Source: CAD feature listing. Evaluate the final solid. Frame: model axes, mm. Give positions to 0.01 mm unless a question says otherwise; leave off trailing zeros. Write each loop counter-clockwise with the first axis right and the second up, starting at its lowest first coordinate (ties: lowest second). Pieces come first, ordered by that corner, then holes. Notation, with made-up numbers: M 56,-5.75 L 114,-5.75 A17 ccw 114,6.25 Z; hole C 63,11.25 d11. An arc over 180 degrees is marked long. Answer as a JSON object with one key per item and string values. Group by question number.
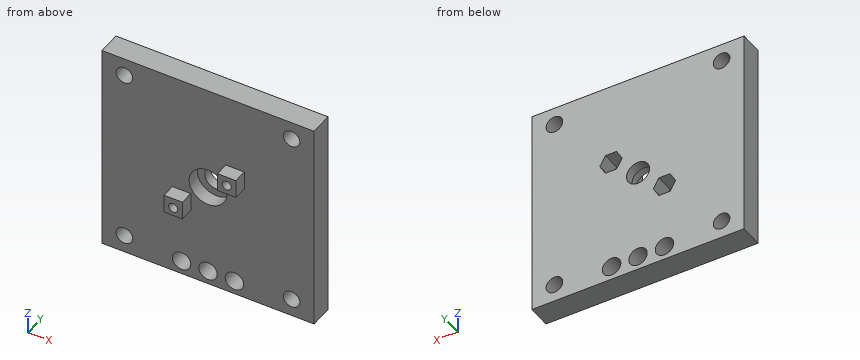
```python
from build123d import *

# Parameters (mm, degrees)
SKETCH2_W           = 46
SKETCH2_H           = 46
BOSS_EXTRUDE1_DEPTH = 5
SKETCH3_R           = 1.8
SKETCH3_R_2         = 2.5
CUT_EXTRUDE1_DEPTH  = 5
SKETCH4_R           = 4.1
CUT_EXTRUDE2_DEPTH  = 3
SKETCH5_W           = 4
SKETCH5_H           = 4
BOSS_EXTRUDE2_DEPTH = 3
SKETCH6_R           = 1
CUT_EXTRUDE3_DEPTH  = 9
CUT_EXTRUDE5_DEPTH  = 4
SKETCH9_R           = 2
CUT_EXTRUDE6_DEPTH  = 6


with BuildPart() as part:
    # Sketch2 → Boss-Extrude1 (new body)
    with BuildSketch(Plane(origin=(0, 0, 0), x_dir=(1, 0, 0), z_dir=(0, 1, 0))):
        Rectangle(SKETCH2_W, SKETCH2_H)
    extrude(amount=BOSS_EXTRUDE1_DEPTH)

    # Sketch3 → Cut-Extrude1 (cut)
    with BuildSketch(Plane(origin=(0, 0, 0), x_dir=(1, 0, 0), z_dir=(0, 1, 0))):
        with Locations((-18.12, 19.125)):
            Circle(SKETCH3_R)
        with Locations((18.12, 19.125)):
            Circle(SKETCH3_R)
        with Locations((18.12, -19.125)):
            Circle(SKETCH3_R)
        with Locations((-18.12, -19.125)):
            Circle(SKETCH3_R)
        Circle(SKETCH3_R_2)
    extrude(amount=CUT_EXTRUDE1_DEPTH, mode=Mode.SUBTRACT)

    # Sketch4 → Cut-Extrude2 (cut)
    with BuildSketch(Plane(origin=(0, 0, 0), x_dir=(1, 0, 0), z_dir=(0, 1, 0))):
        Circle(SKETCH4_R)
    extrude(amount=CUT_EXTRUDE2_DEPTH, mode=Mode.SUBTRACT)

    # Sketch5 → Boss-Extrude2 (add)
    with BuildSketch(Plane(origin=(0, 0, 0), x_dir=(1, 0, 0), z_dir=(0, 1, 0))):
        with Locations((-5.7330026, 5.06948708)):
            Rectangle(SKETCH5_W, SKETCH5_H)
        with Locations((5.862376563, -4.939727226)):
            Rectangle(SKETCH5_W, SKETCH5_H)
    extrude(amount=-BOSS_EXTRUDE2_DEPTH)

    # Sketch6 → Cut-Extrude3 (cut, through all)
    with BuildSketch(Plane(origin=(0, -3, 0), x_dir=(-1, 0, 0), z_dir=(0, -1, 0))):
        with Locations((5.7330026, 5.230811807)):
            Circle(SKETCH6_R)
        with Locations((-5.862376563, -4.939727226)):
            Circle(SKETCH6_R)
    extrude(amount=-CUT_EXTRUDE3_DEPTH, mode=Mode.SUBTRACT)

    # Sketch8 → Cut-Extrude5 (cut)
    with BuildSketch(Plane(origin=(0, 5, 0), x_dir=(1, 0, 0), z_dir=(0, 1, 0))):
        Polygon((8.287247693, -4.939727226), (7.074812128, -2.839727226), (4.649940998, -2.839727226), (3.437505432, -4.939727226), (4.649940998, -7.039727226), (7.074812128, -7.039727226), align=None)
        Polygon((-3.30813147, 5.230811807), (-4.520567035, 7.330811807), (-6.945438166, 7.330811807), (-8.157873731, 5.230811807), (-6.945438166, 3.130811807), (-4.520567035, 3.130811807), align=None)
    extrude(amount=-CUT_EXTRUDE5_DEPTH, mode=Mode.SUBTRACT)

    # Sketch9 → Cut-Extrude6 (cut, through all)
    with BuildSketch(Plane(origin=(0, 0, 0), x_dir=(1, 0, 0), z_dir=(0, 1, 0))):
        with Locations((-5.7330026, 20)):
            Circle(SKETCH9_R)
        with Locations((5.73, 20)):
            Circle(SKETCH9_R)
        with Locations((0, 20)):
            Circle(SKETCH9_R)
    extrude(amount=CUT_EXTRUDE6_DEPTH, mode=Mode.SUBTRACT)


solid = part.part
```
(1) Section D-D, the plane y = 2.25. State how many separate pieces and enclosed holes the cut face has, plus the area to 3 significant figures.
(2) Section C-C, the plane z = -20. Return loops of the section in (x, y), plus the area to 3 significant figures.
(3) Section A-A, the plane y = -1.25. Return loops of the section in (x, z), plus the area to 3 significant figures.
(4) Ray query, L1, parallel to Z at x = 0, y = 3.65; L2, parallel to Z at x = 18.12, y = 1.8 (3 decimals); L3, parallel to X at y = 4.5, z = -20.5. Return the intervals inside material, ascending. Write a range as [from, to].
(5) Section B-B, the plane x = 18.12. Return loops of the section in (y, z) (3 decimals), plus the area to 3 significant figures.
(6) Contact query for flat-ended pins moving along their axis: pin 1 Ø6 at (x, z) = (0, 0) entering from -Y; pin 2 Ø14 at (x, z) = (4.5, -10) entering from -Y; pin 3 Ø0.9 at (y, z) = (-1, -5.5) entering from +X. Output: stop coordinate, or through.
Reported:
{
 "1": {"separate pieces": "1", "enclosed holes": "10", "area": "1,950 mm2"},
 "2": {"outline": "M -23,0 L -19.69,0 L -19.69,5 L -23,5 Z; M -16.55,0 L -7.73,0 L -7.73,5 L -16.55,5 Z; M -3.73,0 L -2,0 L -2,5 L -3.73,5 Z; M 2,0 L 3.73,0 L 3.73,5 L 2,5 Z; M 7.73,0 L 16.55,0 L 16.55,5 L 7.73,5 Z; M 19.69,0 L 23,0 L 23,5 L 19.69,5 Z", "area": "139 mm2"},
 "3": {"outline": "M -7.73,-7.07 L -3.73,-7.07 L -3.73,-3.07 L -7.73,-3.07 Z; M 3.86,2.94 L 7.86,2.94 L 7.86,6.94 L 3.86,6.94 Z; hole C -5.73,-5.23 d2; hole C 5.86,4.94 d2", "area": "25.7 mm2"},
 "4": {"L1": "z = [-23, -22], [-18, -2.5], [2.5, 23]", "L2": "z = [-23, -20.925], [-17.325, 17.325], [20.925, 23]", "L3": "x = [-23, -19.28], [-16.96, -7.67], [-3.8, -1.94], [1.94, 3.79], [7.67, 16.96], [19.28, 23]"},
 "5": {"outline": "M 0,-23 L 5,-23 L 5,-20.925 L 0,-20.925 Z; M 0,-17.325 L 5,-17.325 L 5,17.325 L 0,17.325 Z; M 0,20.925 L 5,20.925 L 5,23 L 0,23 Z", "area": "194 mm2"},
 "6": {"pin 1": "stops at y = 3", "pin 2": "stops at y = 0", "pin 3": "stops at x = -3.73"}
}
